Geometry: see drawing. Coordinates: mm, zero at the bounding-box minimum. Coordinates: 2 decimals unless noted, no trailing zeros. Loops run counter-clockwise (first coordinate to the right, second up) from the corner with the lowest first, then second, coordinate; pieces in that order, holes last. Notation, with made-up numbers: (17.25, 42) - (47.25, 42) arc R17 ccw to (47.25, 54) - close; hole circle Ø9 at (87.5, 12). An arc over 180 degrees is marked (long way). Use a Markdown table: item, result. Add a question column.
1. Section query A-A on x = 9.75. Return the cut outline in (y, z).
2. Section query D-D on z = 12.25. Return the cut outline in (x, y), then the cut area to 3 significant figures.
3. Section query B-B on z = 2.5. Return the cut outline in (x, y).
4. Ray query, L1, parallel to Z at x = 6.5, y = 0.35; L2, parallel to X at y = 0.25, z = 5.5 (1 decimal); L3, parallel to Z at x = 2, y = 2.25 (1 decimal). Return the intervals inside material, ascending. Write a range as [from, to].
5. Contact query for a flat-ended pin moving along its axis: P1, Ø1, axis at x = 9, y = 0.5, coming from the +Z side (1 decimal). Output: stop coordinate, or through.
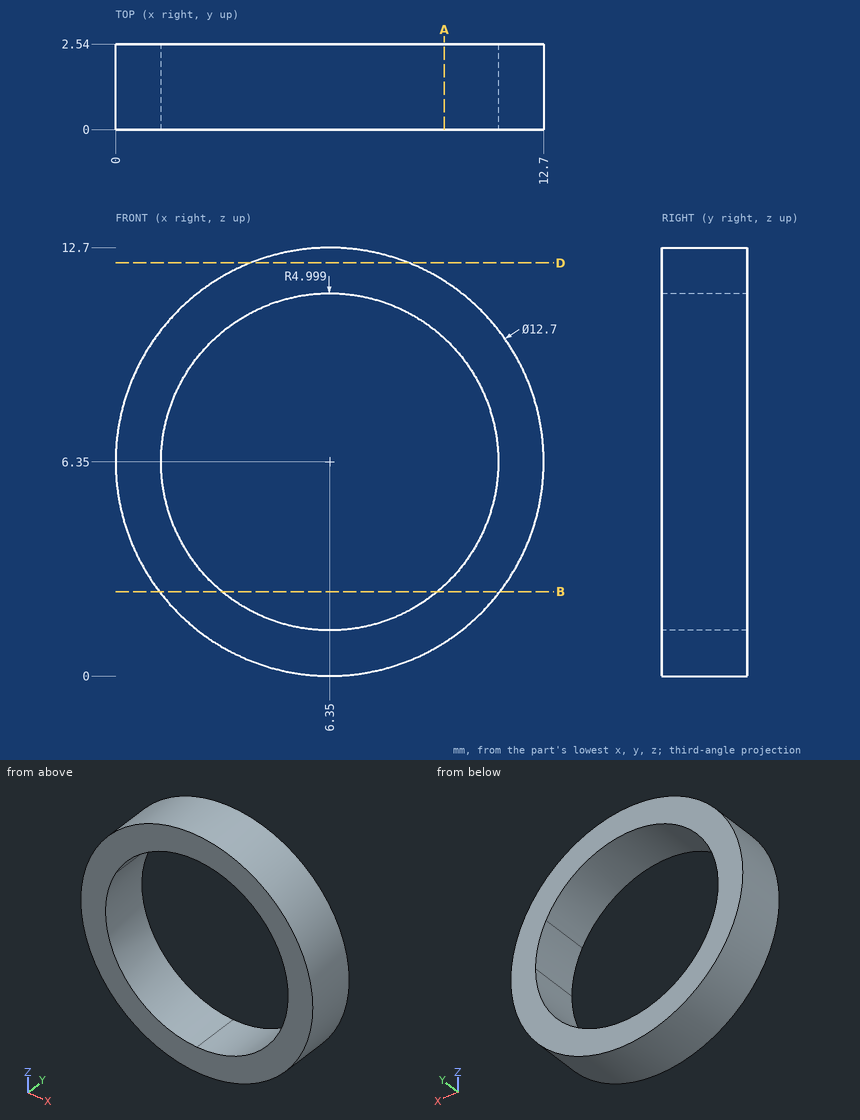
Resolved:
| question | item | result |
|---|---|---|
| 1 | outline | (0, 0.99) - (2.54, 0.99) - (2.54, 2.69) - (0, 2.69) - close; (0, 10.01) - (2.54, 10.01) - (2.54, 11.71) - (0, 11.71) - close |
| 2 | outline | (4, 0) - (8.7, 0) - (8.7, 2.54) - (4, 2.54) - close |
| 2 | area | 11.9 mm² |
| 3 | outline | (1.3, 0) - (3.16, 0) - (3.16, 2.54) - (1.3, 2.54) - close; (9.54, 0) - (11.4, 0) - (11.4, 2.54) - (9.54, 2.54) - close |
| 4 | L1 | [0, 1.35], [11.35, 12.7] |
| 4 | L2 | [0.1, 1.4], [11.3, 12.6] |
| 4 | L3 | [1.7, 3.9], [8.8, 11] |
| 5 | P1 | z = 12.3 |
